Input: part model. Units: mm. Frame: model coordinates. Face numbers are marked on the shaded views. A direction names the side the tool comes from. Give positions to 0.01 mm unless a question says otherwise; leave off trailing zeros. Write each loop counter-clockwise with the first axis right and the second up, starting at its lowest first coordinate (ties: lowest second). Pieces come first, ordered by that corner, then holes. Notation, with made-up numbers: (-24, -16.75) - (13, -16.75) arc R23 cw to (13, -8.75) - close; hole circle Ø4 at (51.25, -5). An arc over 180 degrees is marked (long way). Use a Markdown table: item, result. Add a question column.
1. Pin query (flat end, axial travel): pin 1 (2 mm diameter, centred on x = -354, z = -592.5, fed in from -Y); pin 2 (3 mm diameter, centred on x = -169, z = -38, fed in from +Y). Return the tip coordinate at first contact, or that it passes through.
2. Set-up query: the marked faces 1 and 2. Return all of +Z, -Z, +X, -X, +Y, -Y with unobstructed straight access to the full face (end or side cutting, diameter ignored); none if empty.
3. Mould query, pull axis X, two halves, no side actions, for the marked faces 3, 4 and 5. Classes: released by +X, released by -X, zero draft, split by the parting line, or undercut.
4. Section query A-A, the plane x = -380. Return loops of the section in (y, z), plus the area to 3 significant figures.
5. Material intervals for probe 1 along Y at (x, z) = (-394, -348.5); probe 2 along Y at (x, z) = (-105.5, -763), sorted ascending.
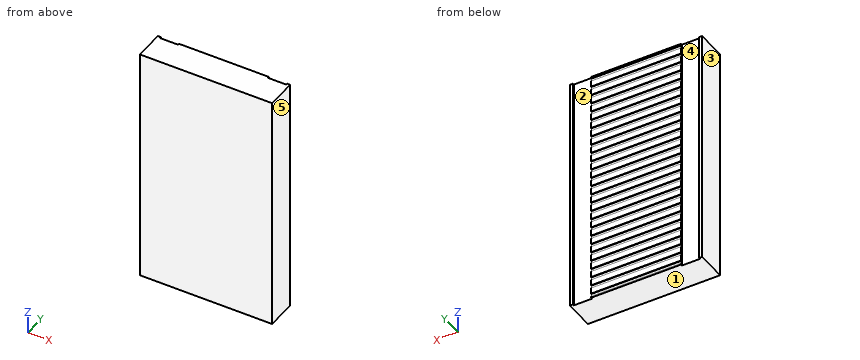
```python
from build123d import *

# Parameters (mm, degrees)
SKETCH_1_W          = 441
SKETCH_1_H          = 800
EXTRUDE_1_DEPTH     = 95
SKETCH_3_W          = 10
SKETCH_3_H          = 800
SKETCH_3_W_2        = 300
EXTRUDE_2_DEPTH     = 5
SKETCH_4_W          = 300
SKETCH_4_H          = 10
CUT_EXTRUDE_1_DEPTH = 2


with BuildPart() as part:
    # 草图1 → 凸台-拉伸1 (new body)
    with BuildSketch(Plane(origin=(0, 0, 0), x_dir=(1, 0, 0), z_dir=(0, 1, 0))):
        with Locations((-220.5, 400)):
            Rectangle(SKETCH_1_W, SKETCH_1_H)
    extrude(amount=EXTRUDE_1_DEPTH)

    # 草图3 → 凸台-拉伸2 (add)
    with BuildSketch(Plane(origin=(0, 95, 0), x_dir=(1, 0, 0), z_dir=(0, 1, 0))):
        with Locations((-436, 400)):
            Rectangle(SKETCH_3_W, SKETCH_3_H)
        with Locations((-220.5, 400)):
            Rectangle(SKETCH_3_W_2, SKETCH_3_H)
        with Locations((-5, 400)):
            Rectangle(SKETCH_3_W, SKETCH_3_H)
    extrude(amount=EXTRUDE_2_DEPTH)

    # 草图4 → 切除-拉伸1 (cut)
    with BuildSketch(Plane(origin=(0, 100, 0), x_dir=(1, 0, 0), z_dir=(0, 1, 0))):
        with Locations((-220.5, 790)):
            Rectangle(SKETCH_4_W, SKETCH_4_H)
        with Locations((-220.5, 760)):
            Rectangle(SKETCH_4_W, SKETCH_4_H)
        with Locations((-220.5, 730)):
            Rectangle(SKETCH_4_W, SKETCH_4_H)
        with Locations((-220.5, 700)):
            Rectangle(SKETCH_4_W, SKETCH_4_H)
        with Locations((-220.5, 670)):
            Rectangle(SKETCH_4_W, SKETCH_4_H)
        with Locations((-220.5, 640)):
            Rectangle(SKETCH_4_W, SKETCH_4_H)
        with Locations((-220.5, 610)):
            Rectangle(SKETCH_4_W, SKETCH_4_H)
        with Locations((-220.5, 580)):
            Rectangle(SKETCH_4_W, SKETCH_4_H)
        with Locations((-220.5, 550)):
            Rectangle(SKETCH_4_W, SKETCH_4_H)
        with Locations((-220.5, 520)):
            Rectangle(SKETCH_4_W, SKETCH_4_H)
        with Locations((-220.5, 490)):
            Rectangle(SKETCH_4_W, SKETCH_4_H)
        with Locations((-220.5, 460)):
            Rectangle(SKETCH_4_W, SKETCH_4_H)
        with Locations((-220.5, 430)):
            Rectangle(SKETCH_4_W, SKETCH_4_H)
        with Locations((-220.5, 400)):
            Rectangle(SKETCH_4_W, SKETCH_4_H)
        with Locations((-220.5, 370)):
            Rectangle(SKETCH_4_W, SKETCH_4_H)
        with Locations((-220.5, 340)):
            Rectangle(SKETCH_4_W, SKETCH_4_H)
        with Locations((-220.5, 310)):
            Rectangle(SKETCH_4_W, SKETCH_4_H)
        with Locations((-220.5, 280)):
            Rectangle(SKETCH_4_W, SKETCH_4_H)
        with Locations((-220.5, 250)):
            Rectangle(SKETCH_4_W, SKETCH_4_H)
        with Locations((-220.5, 220)):
            Rectangle(SKETCH_4_W, SKETCH_4_H)
        with Locations((-220.5, 190)):
            Rectangle(SKETCH_4_W, SKETCH_4_H)
        with Locations((-220.5, 160)):
            Rectangle(SKETCH_4_W, SKETCH_4_H)
        with Locations((-220.5, 130)):
            Rectangle(SKETCH_4_W, SKETCH_4_H)
        with Locations((-220.5, 100)):
            Rectangle(SKETCH_4_W, SKETCH_4_H)
        with Locations((-220.5, 70)):
            Rectangle(SKETCH_4_W, SKETCH_4_H)
        with Locations((-220.5, 40)):
            Rectangle(SKETCH_4_W, SKETCH_4_H)
        with Locations((-220.5, 10)):
            Rectangle(SKETCH_4_W, SKETCH_4_H)
    extrude(amount=-CUT_EXTRUDE_1_DEPTH, mode=Mode.SUBTRACT)


solid = part.part
```
Result sheet:
| question | item | result |
|---|---|---|
| 1 | pin 1 | stops at y = 0 |
| 1 | pin 2 | stops at y = 98 |
| 2 | face 1 | -Z, +X, -X, +Y, -Y |
| 2 | face 2 | +Z, -Z, +Y |
| 3 | face 3 | released by -X |
| 3 | face 4 | undercut |
| 3 | face 5 | released by +X |
| 4 | outline | (0, -800) - (95, -800) - (95, 0) - (0, 0) - close |
| 4 | area | 76,000 mm² |
| 5 | probe 1 | y = 0 to 95 |
| 5 | probe 2 | y = 0 to 98 |
